Autodesk Inventor part; units mm, degrees
sketch "スケッチ1" plane through (0, 0, 0) normal (0, 0, 1) x (1, 0, 0)
  circle A0 centre (0, 0) radius 10.85
  dimension "d0" = 21.7
extrude "押し出し1" add sketch "スケッチ1" along normal blind 1.95
sketch "スケッチ2" plane through (0, 0, 0) normal (0, 0, 1) x (1, 0, 0)
  circle A0 centre (0, 0) radius 4.7
  dimension "d3" = 9.4
extrude "押し出し2" add sketch "スケッチ2" against normal blind 3.5
sketch "スケッチ3" plane through (0, 0, 0) normal (0, 0, 1) x (1, 0, 0)
  circle A0 centre (0, 0) radius 3
  dimension "d6" = 6
extrude "押し出し3" cut sketch "スケッチ3" against normal blind 3.5
sketch "スケッチ4" plane through (0, 0, 0) normal (0, 0, 1) x (1, 0, 0)
  circle A0 centre (0, 0) radius 4.2
  dimension "d9" = 8.4
extrude "押し出し4" add sketch "スケッチ4" along normal blind 2.5
sketch "スケッチ5" plane through (0, 0, 2.5) normal (0, 0, 1) x (1, 0, 0)
  circle A0 centre (0, 0) radius 3.5
  dimension "d12" = 7
extrude "押し出し5" cut sketch "スケッチ5" against normal blind 1.4
sketch "スケッチ6" plane through (0, 0, 0) normal (0, 0, 1) x (1, 0, 0)
  circle A0 centre (0, 0) radius 1.7
  dimension "d15" = 3.4
extrude "押し出し6" cut sketch "スケッチ6" along normal through all
sketch "スケッチ7" plane through (0, 0, 0) normal (0, 0, 1) x (1, 0, 0)
  circle A0 centre (7.8, 0) radius 0.8
  point P0 (0, 0)
  dimension "d18" = 1.6
  dimension "d19" = 7.8
extrude "押し出し7" cut sketch "スケッチ7" along normal through all
pattern_circular "円形状パターン1" count 4 over 360 about axis through (0, 0, -10) along (0, 0, 1) of "押し出し7"
chamfer "面取り1" distance 0.2 angle 45 1 edges at (-4.7, 0, 0)
scale "尺度1" factors (0.8836555, 0.8836555, 0.8836555) then translate (0, 0, 0.2269) bodies 1
properties part number "HbServoHorn01"
The model under review builds one solid part; all positions refer to its coordinate system, in mm. A direction names the side the tool comes from. Round coordinates to 2 decimals unless told otherwise and drop trailing zeros. Loops run counter-clockwise (first coordinate to the right, second up) from the corner with the lowest first, then second, coordinate; pieces in that order, holes last. Notation, with made-up numbers: (50, -38) -> (56, -38) arc R10 ccw to (56, -19) -> close; hole circle Ø11 at (-28.5, -25). An arc over 180 degrees is marked (long way). One line per question, with ' | ' between items. Start each with the question number.
Item 1: Add section D-D, the plane y = -7. Write out the cut boundary in (x, z), then the cut area to 3 significant figures.
Item 2: Draft analysis for pull direction Y (two halves, no side actions). For faces 4 (the face through (-2.104, -1.613, -1.298)), 5 (the face through (-0.6, -7.27, 1.08)), 6 (the face through (0, -4, 1.95)), 7 (the face through (-2.08, 9.36, 1.08)), state which applies: +Y half, -Y half, draft (parallel to the pull), parting line (faces both ways), or undercut.
Item 3: Add section C-C, the plane z = 0.5. Write out the cut boundary in (x, y).
Item 4: For pin 1 (1.5 mm diameter, centred on y = -4.5, z = 1, fed in from +X); pin 2 (1.5 mm diameter, centred on y = -5, z = -2, fed in from -X); pin 3 (4 mm diameter, centred on x = 0, y = 0, fed in from -Z); pin 4 (3 mm diameter, centred on y = 1, z = -2.5, fed in from -X), all flat-tipped, find the tip position at first contact; note any pin that passes through.
Item 5: Add section A-A, the plane y = 0. Count the separate pieces of the cut face and the enclosed holes in it, then the cut area to 3 significant figures.
Item 6: Machinability: for faces 1 (the face through (7.27, -0.6, 1.08)), 2 (the face through (2, 0, 0.227)), 3 (the face through (-0.805, 3.623, 2.19)), which of the approach directions +Z, -Z, +X, -X, +Y, -Y give a long, thin tool a straight path to every point of the face, cutting with its end or side? Answer none if there is none.
Item 7: Wall thickness on line 1 along Y through (x, z) = (0, 0.95); line 2 along Y through (x, z) = (0, 1.4); line 3 along Z through (x, y) = (4.75, -6): over which ranges is each line inside the solid? List them lowest first. Write a range as [from, to].
Return value:
1) outline: (-6.55, 0.23) -> (-0.7, 0.23) -> (-0.7, 1.95) -> (-6.55, 1.95) -> close; (0.7, 0.23) -> (6.55, 0.23) -> (6.55, 1.95) -> (0.7, 1.95) -> close | area: 20.2 mm2
2) face 4: undercut | face 5: undercut | face 6: draft | face 7: parting line
3) outline: circle Ø19.18 at (0, 0); hole circle Ø1.41 at (-6.89, 0); hole circle Ø3 at (0, 0); hole circle Ø1.41 at (0, -6.89); hole circle Ø1.41 at (0, 6.89); hole circle Ø1.41 at (6.89, 0)
4) pin 1: stops at x = 8.82 | pin 2: passes through | pin 3: stops at z = 0.23 | pin 4: stops at x = -4.15
5) separate pieces: 4 | enclosed holes: 0 | area: 30.5 mm2
6) face 1: +Z, -Z | face 2: -Z | face 3: +Z
7) line 1: y = [-9.59, -7.6], [-6.19, -1.5], [1.5, 6.19], [7.6, 9.59] | line 2: y = [-9.59, -7.6], [-6.19, -3.09], [3.09, 6.19], [7.6, 9.59] | line 3: z = [0.23, 1.95]
